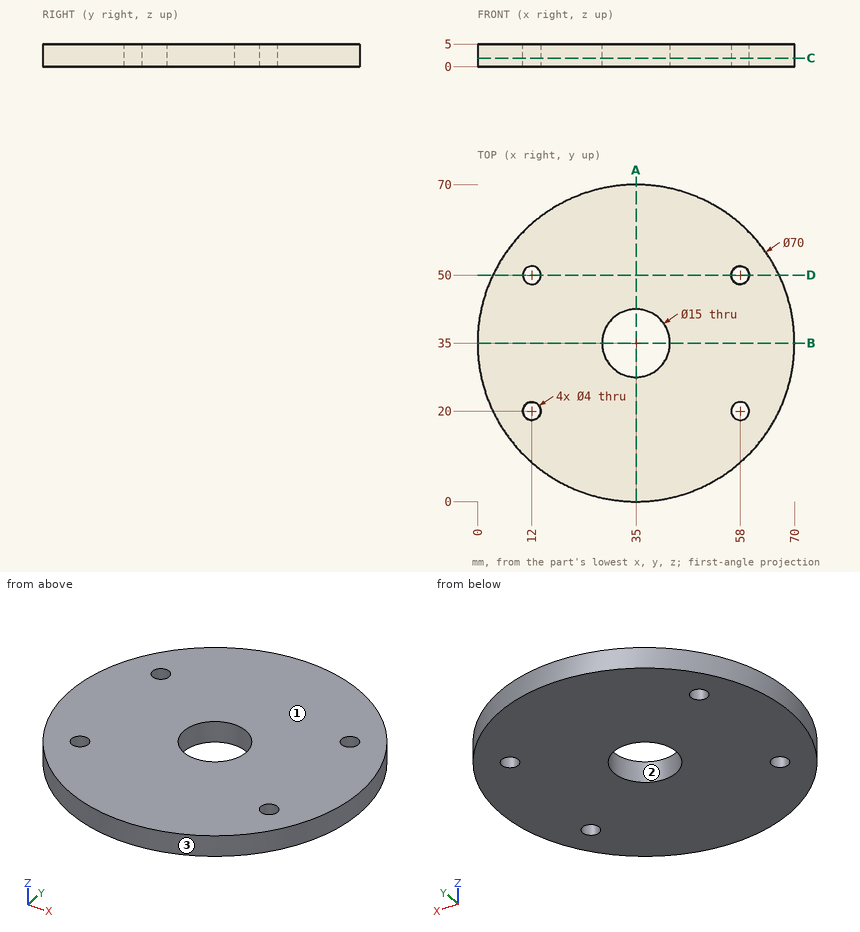
The drawing under review shows one solid part. Ordinate dimensions are in mm from its lowest x, y, z. Round coordinates to 2 decimals unless told otherwise and drop trailing zeros. Write each loop counter-clockwise with the first axis right and the second up, starting at its lowest first coordinate (ties: lowest second). Pieces come first, ordered by that corner, then holes. Notation, with made-up numbers: (-19.5, 18) - (18.5, 18) arc R15 cw to (18.5, 24) - close; hole circle Ø3 at (14.5, 51.25). An arc over 180 degrees is marked (long way). Put each result on its own line as item: value.
Q1. We need section C-C (z = 1.9). Give the boundary of the cut face in (x, y).
Solved:
outline: circle Ø70 at (35, 35); hole circle Ø4 at (12, 20); hole circle Ø4 at (12, 50); hole circle Ø15 at (35, 35); hole circle Ø4 at (58, 20); hole circle Ø4 at (58, 50)
Q2. Wall thickness on probe 1 along Y at (x, z) = (35, 2.25); probe 2 along X at (y, z) = (20, 3.05); probe 3 along X at (y, z) = (51.5, 4): over which ranges is each line inside the solid? List them lowest first.
Solved:
probe 1: y = 0 to 27.5, 42.5 to 70
probe 2: x = 3.38 to 10, 14 to 56, 60 to 66.62
probe 3: x = 4.13 to 10.68, 13.32 to 56.68, 59.32 to 65.87
Q3. Insertion check: pin 1 Ø1.5 at (x, z) = (26, 1.5) entering from -Y; pin 2 Ø1 at (x, z) = (25, 2) entering from +Y; pin 3 Ø3 at (y, z) = (40, 1.5) entering from +X. Each pin has a flat end and moves straight along its axis. Give the tip position at first contact, or say it passes through.
Solved:
pin 1: stops at y = 0.99
pin 2: stops at y = 68.69
pin 3: stops at x = 69.82
Q4. We need section D-D (y = 50). Give the boundary of the cut face in (x, z).
Solved:
outline: (3.38, 0) - (10, 0) - (10, 5) - (3.38, 5) - close; (14, 0) - (56, 0) - (56, 5) - (14, 5) - close; (60, 0) - (66.62, 0) - (66.62, 5) - (60, 5) - close
Q5. We need section A-A (x = 35). Give the boundary of the cut face in (y, z).
Solved:
outline: (0, 0) - (27.5, 0) - (27.5, 5) - (0, 5) - close; (42.5, 0) - (70, 0) - (70, 5) - (42.5, 5) - close
Q6. Mouldability with a two-part tool opening along Y and no side actions: class the marked faces 1, 2 and 3 as released by +Y, released by -Y, zero draft, split by the parting line, or undercut.
Solved:
face 1: zero draft
face 2: undercut
face 3: split by the parting line
